Part print with two shaded views. Sizes in mm from the minimum x, y, z corner. Round coordinates to 2 decimals unless told otherwise and drop trailing zeros. Write each loop counter-clockwise with the first axis right and the second up, starting at its lowest first coordinate (ties: lowest second). Pieces come first, ordered by that corner, then holes.
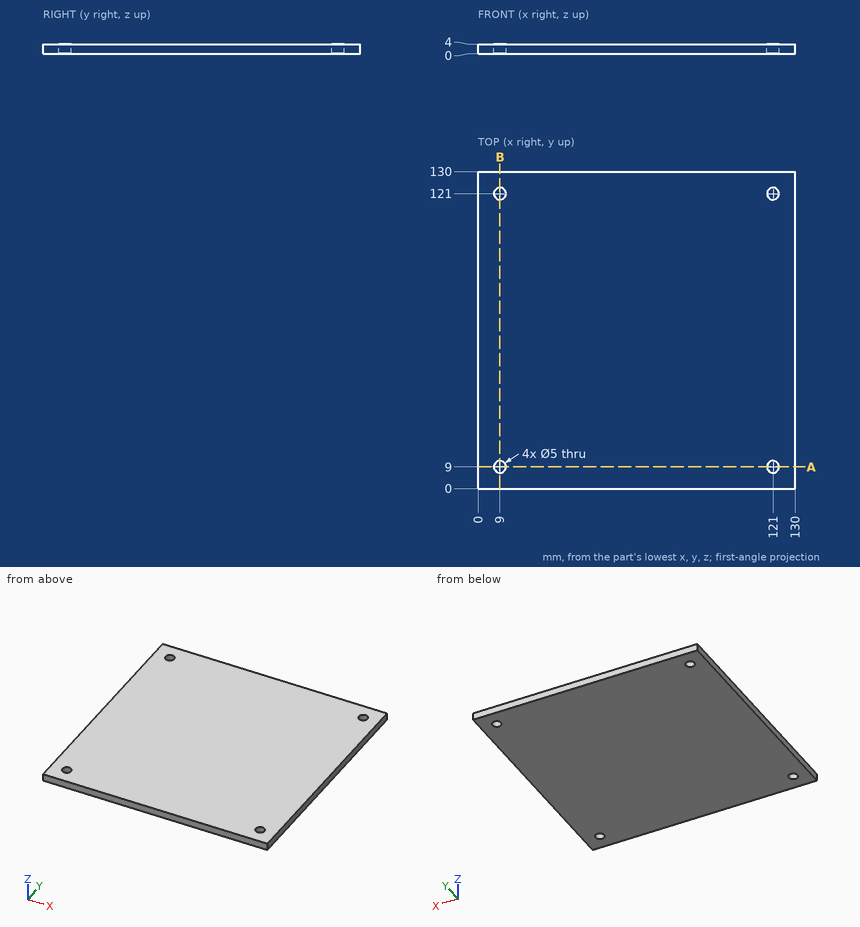
Q1. Drop a flat-ended pin along its axis: pin 1 (4.5 mm diameter, centred on x = 9, y = 121, fed in from +Z). Give the stop position or say it passes through.
Values follow:
pin 1: passes through
Q2. Wall check: L1, parallel to Y at x = 121, z = 1.55. Give the ranges that are in metal, low to high.
Values follow:
L1: y = 0 to 6.5, 11.5 to 118.5, 123.5 to 130
Q3. Cut at A-A on y = 9. Write the cut outline in (x, z).
Values follow:
outline: (0, 0) - (6.5, 0) - (6.5, 4) - (0, 4) - close; (11.5, 0) - (118.5, 0) - (118.5, 4) - (11.5, 4) - close; (123.5, 0) - (130, 0) - (130, 4) - (123.5, 4) - close
